Answer from the drawing. Dimensions are ordinates in mm from the lowest x, y and z of the part. Round coordinates to 2 decimals unless told otherwise and drop trailing zeros. Write each loop counter-clockwise with the first axis right and the second up, starting at its lowest first coordinate (ties: lowest second). Pieces come first, ordered by that corner, then holes. Notation, with made-up numbers: M 20,-7.75 L 69,-7.75 A18 ccw 69,7.25 Z; hole C 41,73.25 d9. An arc over 180 degrees is marked long. Answer as CSV lines item,"result". Start each with the question number.
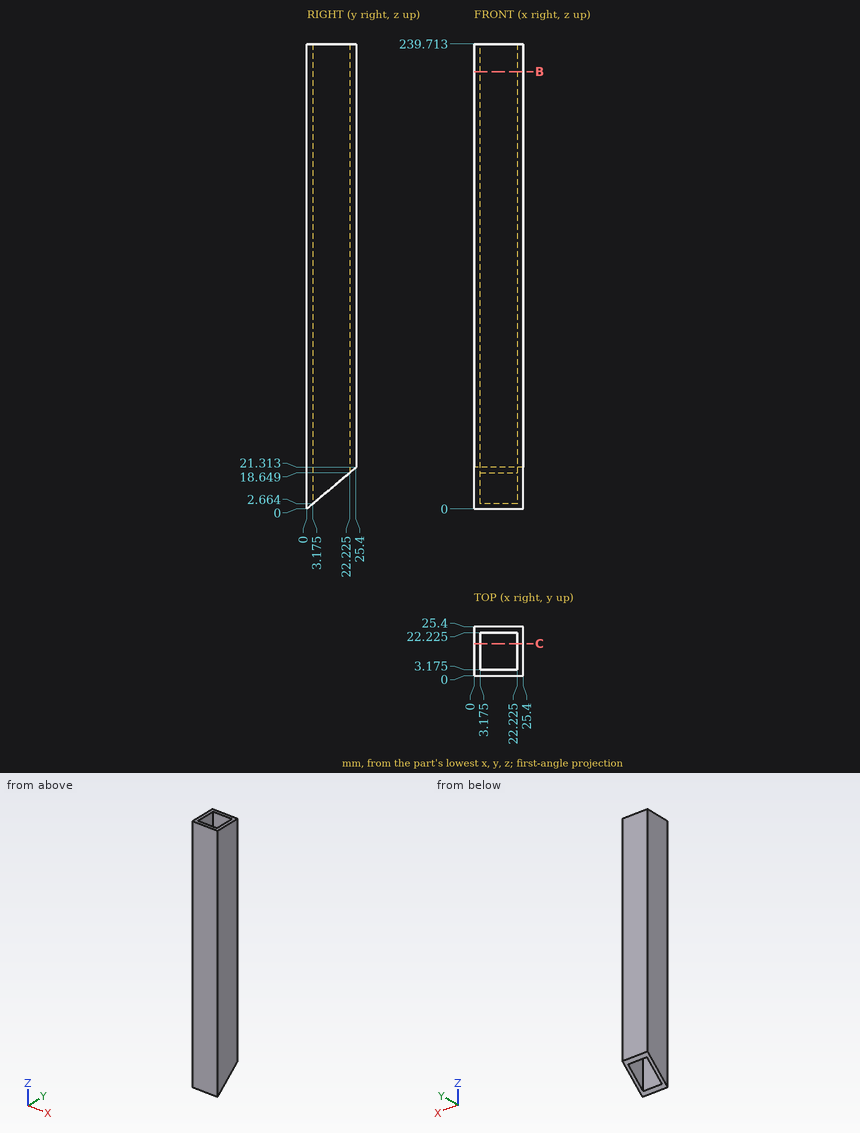
Q1. Find section B-B (z = 225.5). Determine the outline of the cut face in (x, y) (1 decimal), plus the area to 3 significant figures.
Q2. Straight lines are drawn through the part: L1, parallel to X at y = 17.75, z = 124 (1 decimal); L2, parallel to Z at x = 9.5, y = 22.75 (1 decimal). For each, find the intervals that lie inside material, in ascending order.
Q3. This flat-tipped pin is pushed along its axis until it touches: P1, Ø12, axis at x = 5.5, y = 11.5, coming from the -Z side. Where does it stop, or does it pass through?
Q4. Find section C-C (y = 16.75). Determine the outline of the cut face in (x, z) (1 decimal), plus the area to 3 significant figures.
Reported:
1,outline,"M 0,0 L 25.4,0 L 25.4,25.4 L 0,25.4 Z; hole M 3.2,3.2 L 22.2,3.2 L 22.2,22.2 L 3.2,22.2 Z"
1,area,"282 mm2"
2,L1,"x = 0 to 3.2, 22.2 to 25.4"
2,L2,"z = 19.1 to 239.7"
3,P1,"stops at z = 5.01"
4,outline,"M 0,14.1 L 3.2,14.1 L 3.2,239.7 L 0,239.7 Z; M 22.2,14.1 L 25.4,14.1 L 25.4,239.7 L 22.2,239.7 Z"
4,area,"1,430 mm2"
